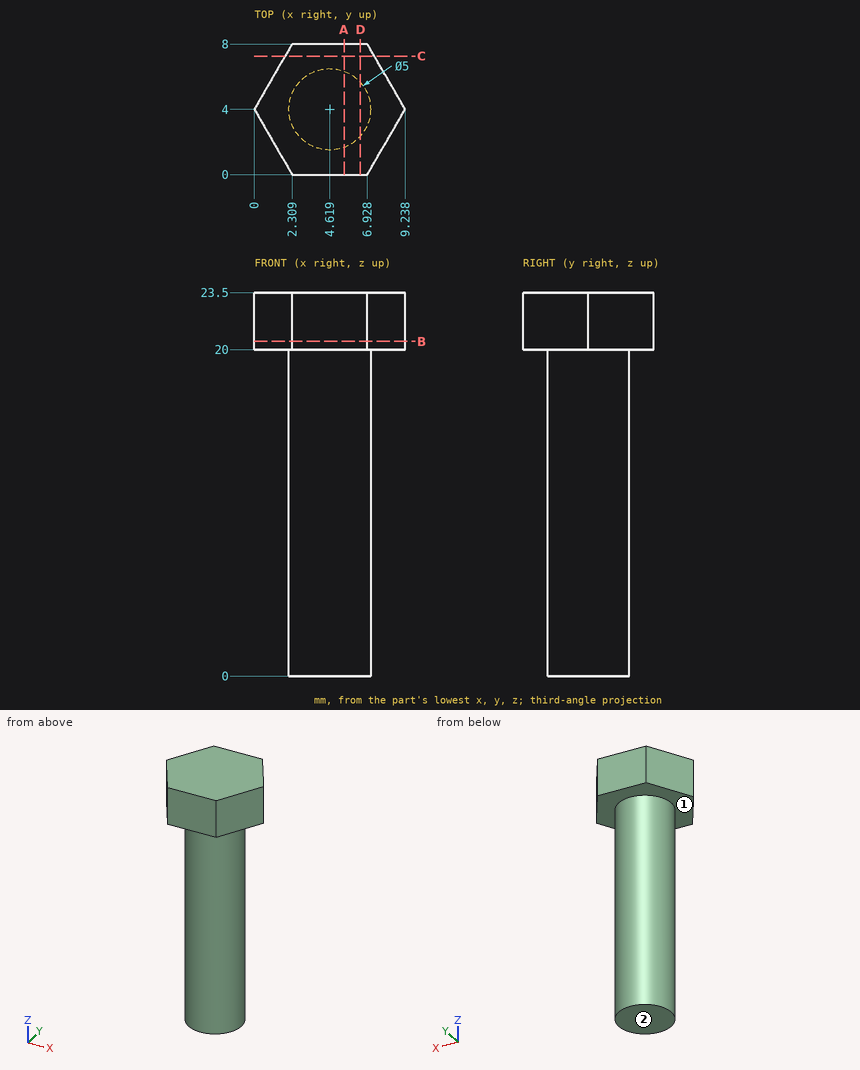
Design review of the part shown in the three views and the two pictorial views. Dimensions are in mm from the part's minimum x, y and z. A direction names the side the tool comes from. Round coordinates to 2 decimals unless told otherwise and drop trailing zeros. Write each loop counter-clockwise with the first axis right and the second up, starting at its lowest first coordinate (ties: lowest second). Pieces come first, ordered by that corner, then holes.
Item 1: Wall thickness on L1, parallel to Z at x = 8.75, y = 3.5; L2, parallel to Y at x = 4.5, z = 17; L3, parallel to X at y = 4, z = 17: over which ranges is each line inside the solid? List them lowest first.
Item 2: Consider section D-D on x = 6.5. Give the boundary of the cut face in (y, z).
Item 3: Consider section C-C on y = 7.25. Give the boundary of the cut face in (x, z), and give its area (3 significant figures).
Item 4: For the marked faces 1 and 2, list the 3-axis set-ups (+Z, -Z, +X, -X, +Y, -Y) from which the entire face can be reached by the end or side of a thin tool; tool diameter is ignored.
Item 5: Consider section B-B on z = 20.5. Give the boundary of the cut face in (x, y), and give its area (3 significant figures).
Item 6: Consider section A-A on x = 5.5. Give the boundary of the cut face in (y, z), and give its area (3 significant figures).
Item 7: For pin 1 Ø3 at (y, z) = (5.5, 8.5) entering from +X; pin 2 Ø1.5 at (y, z) = (6, 12.5) entering from +X; pin 3 Ø1.5 at (y, z) = (2.5, 17) entering from +X, all flat-tipped, find the tip position at first contact; note any pin that passes through.
Check values:
1. L1: z = 20 to 23.5
1. L2: y = 1.5 to 6.5
1. L3: x = 2.12 to 7.12
2. outline: (0, 20) - (2.35, 20) - (2.35, 0) - (5.65, 0) - (5.65, 20) - (8, 20) - (8, 23.5) - (0, 23.5) - close
3. outline: (1.88, 20) - (7.36, 20) - (7.36, 23.5) - (1.88, 23.5) - close
3. area: 19.2 mm2
4. face 1: -Z
4. face 2: -Z, +X, -X, +Y, -Y
5. outline: (0, 4) - (2.31, 0) - (6.93, 0) - (9.24, 4) - (6.93, 8) - (2.31, 8) - close
5. area: 55.4 mm2
6. outline: (0, 20) - (1.66, 20) - (1.66, 0) - (6.34, 0) - (6.34, 20) - (8, 20) - (8, 23.5) - (0, 23.5) - close
6. area: 122 mm2
7. pin 1: stops at x = 7.12
7. pin 2: stops at x = 6.78
7. pin 3: stops at x = 7
